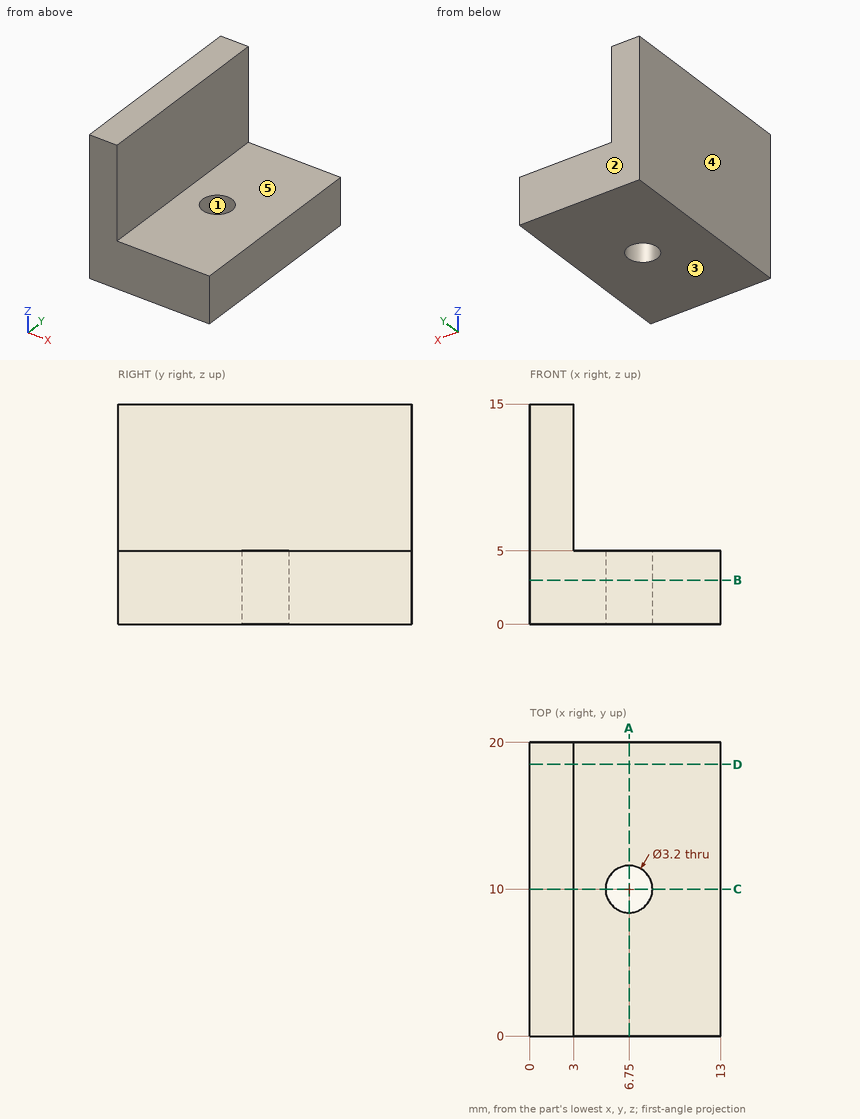
Check sheet for the drawn part. Datum: minimum x, y, z corner. Units: mm. A direction names the side the tool comes from. Round coordinates to 2 decimals unless told otherwise and drop trailing zeros. Loops run counter-clockwise (first coordinate to the right, second up) from the corner with the lowest first, then second, coordinate; pieces in that order, holes last.
Item 1: Gauge pin test, flat ends, axial feed: pin 1 (5 mm diameter, centred on x = 8, y = 15, fed in from +Z); pin 2 (8 mm diameter, centred on y = 5.5, z = 11.5, fed in from +X). Record the tip position at first contact, or that the pin passes through.
Item 2: Cross-section at C-C on y = 10. Record the boundary of the cut face in (x, z).
Item 3: Access from +Z, -Z, +X, -X, +Y, -Y to the whole of each face (thin tool, end or side, straight path). Record for the marked faces 4 and 5.
Item 4: Cross-section at B-B on z = 3. Record the boundary of the cut face in (x, y), then the cut area to 3 significant figures.
Item 5: Thickness scan on line 1 (Y direction, x = 6.75, z = 2.1); line 2 (X direction, y = 14.25, z = 11.5); line 3 (Z direction, x = 10.25, y = 7.5). Record the ranges inside material, lowest first.
Item 6: Cross-section at D-D on y = 18.5. Record the boundary of the cut face in (x, z).
Item 7: Cross-section at A-A on x = 6.75. Record the boundary of the cut face in (y, z), then the cut area to 3 significant figures.
Item 8: Mould release check, pull along Y, two halves, no side actions. Record for the marked faces 1, 2 and 3: pulls with the +Y half, pulls with the -Y half, needs draft (parallel to the pull), parting line crosses it, or undercut.
Answer sheet:
1. pin 1: stops at z = 5
1. pin 2: stops at x = 3
2. outline: (0, 0) - (5.15, 0) - (5.15, 5) - (3, 5) - (3, 15) - (0, 15) - close; (8.35, 0) - (13, 0) - (13, 5) - (8.35, 5) - close
3. face 4: +Z, -Z, -X, +Y, -Y
3. face 5: +Z, +X, +Y, -Y
4. outline: (0, 0) - (13, 0) - (13, 20) - (0, 20) - close; hole circle Ø3.2 at (6.75, 10)
4. area: 252 mm2
5. line 1: y = 0 to 8.4, 11.6 to 20
5. line 2: x = 0 to 3
5. line 3: z = 0 to 5
6. outline: (0, 0) - (13, 0) - (13, 5) - (3, 5) - (3, 15) - (0, 15) - close
7. outline: (0, 0) - (8.4, 0) - (8.4, 5) - (0, 5) - close; (11.6, 0) - (20, 0) - (20, 5) - (11.6, 5) - close
7. area: 84.0 mm2
8. face 1: undercut
8. face 2: pulls with the +Y half
8. face 3: needs draft
